CAD build for the part. Positions are in the model's coordinates, mm. Face numbers are marked on the shaded views. A direction names the side the tool comes from. Round coordinates to 2 decimals unless told otherwise and drop trailing zeros. Order: outer loops, then holes, each group sorted by start corner. A loop starts at its lowest first (then second) coordinate and runs counter-clockwise, first axis right, second up.
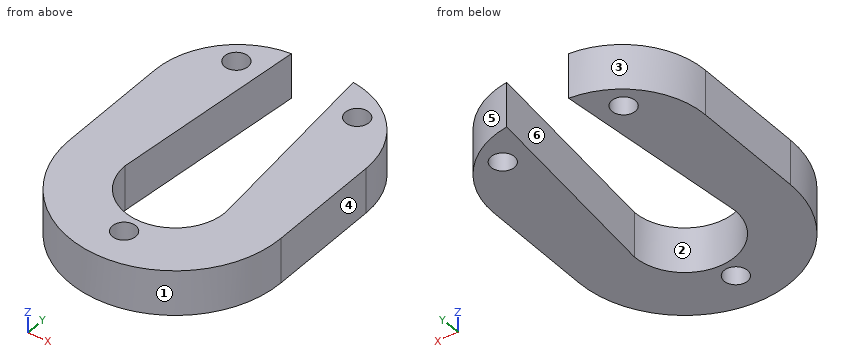
```python
from build123d import *

# Parameters (mm, degrees)
DODANIE_WYCI_GNI_CIE1_DEPTH = 6
SZKIC3_R                    = 1.55
WYTNIJ_WYCI_GNI_CIE2_DEPTH  = 6
SZKIC4_R                    = 1.55
WYTNIJ_WYCI_GNI_CIE3_DEPTH  = 6
WYTNIJ_WYCI_GNI_CIE4_DEPTH  = 6


with BuildPart() as part:
    # Szkic1 → Dodanie-wyciągnięcie1 (new body)
    with BuildSketch(Plane.XY):
        with BuildLine():
            Line((-174.181077779, 72.924846477), (-174.181077779, 87.924846477))
            ThreePointArc((-174.181077779, 87.924846477), (-177.402903186, 95.70302107), (-185.181077779, 98.924846477))
            Line((-185.181077779, 98.924846477), (-191.181077779, 98.924846477))
            ThreePointArc((-191.181077779, 98.924846477), (-198.959252372, 95.70302107), (-202.181077779, 87.924846477))
            Line((-202.181077779, 87.924846477), (-202.181077779, 72.924846477))
            ThreePointArc((-202.181077779, 72.924846477), (-188.181077779, 58.924846477), (-174.181077779, 72.924846477))
        make_face()
    extrude(amount=-DODANIE_WYCI_GNI_CIE1_DEPTH)

    # Szkic3 → Wytnij-wyciągnięcie2 (cut)
    with BuildSketch(Plane.XY):
        with Locations((-196.181077779, 94.324819795)):
            Circle(SZKIC3_R)
        with Locations((-180.181077779, 94.324819795)):
            Circle(SZKIC3_R)
        with Locations((-188.181077779, 63.924846477)):
            Circle(SZKIC3_R)
    extrude(amount=-WYTNIJ_WYCI_GNI_CIE2_DEPTH, mode=Mode.SUBTRACT)

    # Szkic4 → Wytnij-wyciągnięcie3 (cut)
    with BuildSketch(Plane.XY):
        with Locations((-188.181077779, 72.924846477)):
            Circle(SZKIC4_R)
    extrude(amount=-WYTNIJ_WYCI_GNI_CIE3_DEPTH, mode=Mode.SUBTRACT)

    # Szkic7 → Wytnij-wyciągnięcie4 (cut)
    with BuildSketch(Plane(origin=(0, 0, -6), x_dir=(-1, 0, 0), z_dir=(0, 0, -1))):
        with BuildLine():
            Line((181.531097956, 72.941227743), (184.470707897, 102.337327159))
            ThreePointArc((184.470707897, 102.337327159), (188.225739241, 106.074816392), (191.97068627, 102.327222776))
            Line((191.97068627, 102.327222776), (194.831077602, 72.923309279))
            ThreePointArc((194.831077602, 72.923309279), (188.172118542, 66.274852512), (181.531097956, 72.941227743))
        make_face()
    extrude(amount=-WYTNIJ_WYCI_GNI_CIE4_DEPTH, mode=Mode.SUBTRACT)


solid = part.part
```
1. Cut at D-D, the plane x = -200.25. Write the cut outline in (y, z).
2. Tool access for the marked faces 5 and 6: list every direction of +Z, -Z, +X, -X, +Y, -Y with a clear straight run to the whole face (end or side of a thin tool).
3. Pin check, flat tips, straight feed: P1, Ø4, axis at x = -180.18, y = 94.32, coming from the +Z side; P2, Ø1.5, axis at y = 70, z = -5, coming from the +X side; P3, Ø3, axis at x = -191, y = 88.5, coming from the +Z side; P4, Ø1.5, axis at x = -181, z = -4, coming from the +Y side. Stop position of each tip, or through.
4. Cut at B-B, the plane z = -5.3. Write the cut outline in (x, y).
5. Cut at C-C, the plane x = -196.25. Write the cut outline in (y, z), and give its area (3 significant figures).
6. Drill centre lines: line 1 (X direction, y = 94, z = -3.85); line 2 (X direction, y = 94.5, z = -1.75); line 3 (X direction, y = 81, z = -3.05). Where is each one in solid material? Low to high.
7. Mould opens along X. For the marked faces 1, 2, 3 and 4 say: released by +X, released by -X, zero draft, split by the parting line, or undercut.
8. Cut at A-A, the plane y = 92. Write the cut outline in (x, z), and give its area (3 significant figures).
Outcome:
1. outline: (65.83, -6) - (94.15, -6) - (94.15, 0) - (65.83, 0) - close
2. face 5: +Z, -Z, +X, +Y
2. face 6: +Z, -Z
3. P1: stops at z = 0
3. P2: stops at x = -174.35
3. P3: passes through
3. P4: stops at y = 98.38
4. outline: (-202.18, 72.92) arc R14 ccw to (-174.18, 72.92) - (-174.18, 87.92) arc R11 ccw to (-184.12, 98.87) - (-181.53, 72.94) arc R6.65 cw to (-194.83, 72.92) - (-192.31, 98.87) arc R11 ccw to (-202.18, 87.92) - close; hole circle Ø3.1 at (-196.18, 94.32); hole circle Ø3.1 at (-188.18, 63.92); hole circle Ø3.1 at (-180.18, 94.32)
5. outline: (61.48, -6) - (92.78, -6) - (92.78, 0) - (61.48, 0) - close; (95.87, -6) - (97.69, -6) - (97.69, 0) - (95.87, 0) - close
5. area: 199 mm2
6. line 1: x = -200.35 to -197.7, -194.67 to -192.78, -183.64 to -181.7, -178.67 to -176.01
6. line 2: x = -200 to -197.72, -194.64 to -192.73, -183.69 to -181.72, -178.64 to -176.36
6. line 3: x = -202.18 to -194.05, -182.34 to -174.18
7. face 1: split by the parting line
7. face 2: undercut
7. face 3: released by -X
7. face 4: released by +X
8. outline: (-201.4, -6) - (-192.98, -6) - (-192.98, 0) - (-201.4, 0) - close; (-183.44, -6) - (-174.96, -6) - (-174.96, 0) - (-183.44, 0) - close
8. area: 101 mm2
